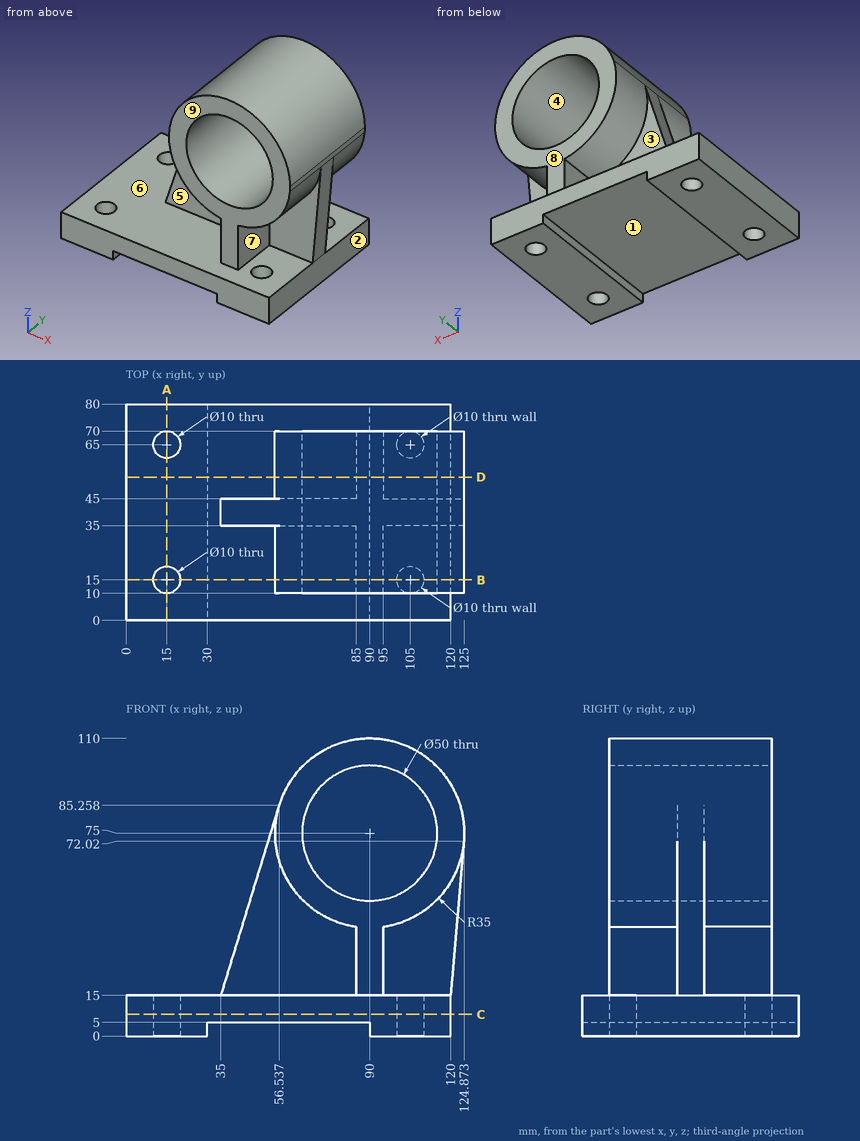
Answer from the drawing. Dimensions are ordinates in mm from the lowest x, y and z of the part. A direction names the side the tool comes from. Give positions to 0.01 mm unless a question says otherwise; leave off trailing zeros. Loops run counter-clockwise (first coordinate to the right, second up) from the corner with the lowest first, then second, coordinate; pieces in that order, holes last. Notation, with made-up numbers: M 42,69 L 91,69 A31 cw 91,105 Z; hole C 41,2 d8. An arc over 180 degrees is marked long. One line per item, written item: value.
Q1. A cutting plane is placed at A-A on x = 15. Determine the outline of the cut face in (y, z).
Working result:
outline: M 0,0 L 10,0 L 10,15 L 0,15 Z; M 20,0 L 60,0 L 60,15 L 20,15 Z; M 70,0 L 80,0 L 80,15 L 70,15 Z
Q2. Flat-ended cylindrical pins translate along their axes: P1, Ø21, axis at x = 104.5, z = 73.5, coming from the +Y side; P2, Ø4, axis at y = 24, z = 3.5, coming from the +X side; P3, Ø8, axis at x = 105, y = 15, coming from the +Z side. Find the tip coordinate at first contact, or state that the pin passes through.
Working result:
P1: stops at y = 70
P2: stops at x = 120
P3: stops at z = 108.23
Q3. A cutting plane is placed at D-D on y = 53. Determine the outline of the cut face in (x, z), then the cut area to 3 significant figures.
Working result:
outline: M 0,0 L 30,0 L 30,5 L 90,5 L 90,0 L 120,0 L 120,15 L 95,15 L 95,40.36 A35 ccw long 85,40.36 L 85,15 L 0,15 Z; hole C 90,75 d50
area: 3,640 mm^2
Q4. Determine the mould class of the marked faces 1, 2, 3 and 4 for opening direction Z: +Z half, -Z half, draft (parallel to the pull), parting line (faces both ways), or undercut.
Working result:
face 1: -Z half
face 2: draft
face 3: undercut
face 4: undercut
Q5. A cutting plane is placed at C-C on z = 8. Determine the outline of the cut face in (x, y).
Working result:
outline: M 0,0 L 120,0 L 120,80 L 0,80 Z; hole C 15,15 d10; hole C 15,65 d10; hole C 105,15 d10; hole C 105,65 d10
Q6. A cutting plane is placed at B-B on y = 15. Determine the outline of the cut face in (x, z), then the cut area to 3 significant figures.
Working result:
outline: M 0,0 L 10,0 L 10,15 L 0,15 Z; M 20,0 L 30,0 L 30,5 L 90,5 L 90,0 L 100,0 L 100,15 L 95,15 L 95,40.36 A35 ccw long 85,40.36 L 85,15 L 20,15 Z; M 110,0 L 120,0 L 120,15 L 110,15 Z; hole C 90,75 d50
area: 3,340 mm^2
Q7. Find the intervals of material crossed by line 1 (Y direction, x = 105, z = 4.25); line 2 (Z direction, x = 69.5, y = 27); line 3 (Z direction, x = 113, y = 58.5), in increasing order. Write a range as from..to.
Working result:
line 1: y = 0..10, 20..60, 70..80
line 2: z = 5..15, 46.63..60.69, 89.31..103.37
line 3: z = 0..15, 48.62..65.2, 84.8..101.38
Q8. For the marked faces 5, 6, 7, 8 and 9, determine the directions among +Z, -Z, +X, -X, +Y, -Y from which every point of the face is accessible in a straight line to the end or side of a thin tool.
Working result:
face 5: -X, -Y
face 6: none
face 7: +X, -Y
face 8: +Z, +X, -X, +Y
face 9: +Z, +X, -X, -Y
